from build123d import *

# Parameters (mm, degrees)
SKETCH1_R           = 5
BOSS_EXTRUDE1_DEPTH = 13
FILLET2_R           = 1
SKETCH2_R           = 4
BOSS_EXTRUDE2_DEPTH = 7


with BuildPart() as part:
    # Sketch1 → Boss-Extrude1 (new body)
    with BuildSketch(Plane(origin=(0, 0, 0), x_dir=(1, 0, 0), z_dir=(0, 1, 0))):
        with Locations(Location((0, 0, 0), (0, 0, 90))):
            Circle(SKETCH1_R)
    extrude(amount=BOSS_EXTRUDE1_DEPTH)

    # Fillet2
    fillet2_edges = [part.edges().sort_by_distance(p)[0] for p in [
        (0, 0, 5),
    ]]
    fillet(fillet2_edges, radius=FILLET2_R)

    # Sketch2 → Boss-Extrude2 (add)
    with BuildSketch(Plane(origin=(0, 13, 0), x_dir=(1, 0, 0), z_dir=(0, 1, 0))):
        with Locations(Location((0, 0, 0), (0, 0, 270))):
            Circle(SKETCH2_R)
    extrude(amount=BOSS_EXTRUDE2_DEPTH)


solid = part.part
The listing builds one solid part. Answer for the finished solid, in the listing's coordinates (mm). A direction names the side the tool comes from. Give positions to 0.01 mm unless a question says otherwise; leave off trailing zeros. Order: outer loops, then holes, each group sorted by start corner. A loop starts at its lowest first (then second) coordinate and runs counter-clockwise, first axis right, second up. Notation, with made-up numbers: (-6.5, 54) -> (51.5, 54) arc R19 cw to (51.5, 89) -> close; hole circle Ø7 at (48, 45). An arc over 180 degrees is marked (long way). Put each result on its own line as item: value.
Item 1: A cutting plane is placed at A-A on z = 0. Give the vertices of the cut face in (x, y), plus the area to 3 significant figures.
Established:
outline: (-5, 1) arc R1 ccw to (-4, 0) -> (4, 0) arc R1 ccw to (5, 1) -> (5, 13) -> (4, 13) -> (4, 20) -> (-4, 20) -> (-4, 13) -> (-5, 13) -> close
area: 186 mm^2
Item 2: Straight lines are drawn through the part: line 1 (Z direction, x = 3, y = 11); line 2 (Y direction, x = 2.5, z = -3.25); line 3 (X direction, y = 7, z = 2.25). For each, find the intervals that lie inside material, in ascending order.
Established:
line 1: z = -4 to 4
line 2: y = 0.01 to 13
line 3: x = -4.47 to 4.47
Item 3: Given P1, Ø1.5, axis at x = 1.5, y = 16, coming from the -Z side; P2, Ø1, axis at y = 7, z = 2, coming from the -X side; P3, Ø4, axis at y = 17, z = -3.5, coming from the +X side, each flat-ended and moving along its own axis, determine where each tip first touches the part or whether it passes through.
Established:
P1: stops at z = -3.93
P2: stops at x = -4.77
P3: stops at x = 3.71
Item 4: A cutting plane is placed at C-C on y = 2. Give the vertices of the cut face in (x, z), plus the area to 3 significant figures.
Established:
outline: circle Ø10 at (0, 0)
area: 78.5 mm^2
Item 5: A cutting plane is placed at B-B on x = 0. Give the vertices of the cut face in (y, z), plus the area to 3 significant figures.
Established:
outline: (0, -4) arc R1 ccw to (1, -5) -> (13, -5) -> (13, -4) -> (20, -4) -> (20, 4) -> (13, 4) -> (13, 5) -> (1, 5) arc R1 ccw to (0, 4) -> close
area: 186 mm^2
Item 6: For faces 1 (the face through (-3.905, 16.451, -0.867)), 2 (the face through (4.88, 6.92, 1.08)), determine the directions among +Z, -Z, +X, -X, +Y, -Y from which every point of the face is accessible in a straight line to the end or side of a thin tool.
Established:
face 1: +Y
face 2: +Y, -Y
